from build123d import *

# Parameters (mm, degrees)
F0_R     = 47.2126506678
F0_R_2   = 20.2272154061
F1_DEPTH = 50.8
F2_R     = 3.175
F2_R_2   = 4.8238037601
F3_DEPTH = 50.801
F4_R     = 4.3834323194
F5_ANGLE = 180


# Not quite as in the source:
# - the program builds the solid bodies; features that only make, move or delete a surface that nothing else refers to are left out


with BuildPart() as f1:
    # F0 (on Front) → F1 (new body)
    with BuildSketch(Plane.XZ):
        Circle(F0_R)
        Circle(F0_R_2, mode=Mode.SUBTRACT)
    extrude(amount=F1_DEPTH)

    # F2 (on Front) → F3 (cut, through all)
    with BuildSketch(Plane.XZ):
        with Locations((0, 34.7616262734)):
            Circle(F2_R)
        with Locations((0, -35.3442244232)):
            Circle(F2_R_2)
    extrude(amount=F3_DEPTH, mode=Mode.SUBTRACT)

    # F4 (on Front) → F5 (revolve)
    with BuildSketch(Plane.XZ):
        with Locations((-34.811783582, 0)):
            Circle(F4_R)
    revolve(axis=Axis((0, 0, 1.5608235262), (0, 0, -1)), revolution_arc=F5_ANGLE)


solid = f1.part
Geometry check sheet. Reference: the model listing, model coordinates, mm. Round coordinates to 2 decimals unless told otherwise and drop trailing zeros. Write each loop counter-clockwise with the first axis right and the second up, starting at its lowest first coordinate (ties: lowest second). Pieces come first, ordered by that corner, then holes.
Item 1: Section check D-D (y = -36.5). Record the boundary of the cut face in (x, z) (3 decimals), plus the area to 3 significant figures.
Determined:
outline: circle Ø94.425 at (0, 0); hole circle Ø40.454 at (0, 0); hole circle Ø9.648 at (0, -35.344); hole circle Ø6.35 at (0, 34.762)
area: 5,610 mm2
Item 2: Section check A-A (z = -33). Record the boundary of the cut face in (x, y).
Determined:
outline: (-33.76, -50.8) - (-4.22, -50.8) - (-4.22, 0) - (-33.76, 0) - close; (4.22, -50.8) - (33.76, -50.8) - (33.76, 0) - (4.22, 0) - close
Item 3: Section check C-C (z = -16.5). Record the boundary of the cut face in (x, y), plus the area to 3 significant figures.
Determined:
outline: (-44.24, -50.8) - (-11.7, -50.8) - (-11.7, 0) - (-44.24, 0) - close; (11.7, -50.8) - (44.24, -50.8) - (44.24, 0) - (11.7, 0) - close
area: 3,310 mm2
Item 4: Go/stop test with flat-tipped pins: pin 1 Ø1.5 at (x, z) = (-20.5, 31) entering from +Y; pin 2 Ø2 at (y, z) = (-27, 8) entering from +X; pin 3 Ø4 at (y, z) = (-10, 25.5) entering from -X; pin 4 Ø12.5 at (x, z) = (0, -35.34) entering from -Y. Record where each tip stops, or that it passes through.
Determined:
pin 1: stops at y = 0
pin 2: stops at x = 46.69
pin 3: stops at x = -40.95
pin 4: stops at y = -50.8
Item 5: Material ranges on line 1 along Z through (x, y) = (0, -12); line 2 along Z through (x, y) = (2, -17); line 3 along Y through (x, z) = (-28, 34), recorded low to high.
Determined:
line 1: z = -47.21 to -40.17, -30.52 to -20.23, 20.23 to 31.59, 37.94 to 47.21
line 2: z = -47.17 to -39.73, -30.95 to -20.13, 20.13 to 32.3, 37.23 to 47.17
line 3: y = -50.8 to 0
Item 6: Section check B-B (x = 0). Record the boundary of the cut face in (y, z), plus the area to 3 significant figures.
Determined:
outline: (-50.8, -47.21) - (0, -47.21) - (0, -40.17) - (-50.8, -40.17) - close; (-50.8, -30.52) - (0, -30.52) - (0, -20.23) - (-50.8, -20.23) - close; (-50.8, 20.23) - (0, 20.23) - (0, 31.59) - (-50.8, 31.59) - close; (-50.8, 37.94) - (0, 37.94) - (0, 47.21) - (-50.8, 47.21) - close; circle Ø8.77 at (34.81, 0)
area: 1,990 mm2
Item 7: Mould release check, pull along X, two halves, no side actions. Record for faces 1 (the face through (10, -50.8, -20)), 2 (the face through (-4.385, -25.044, -19.746)), 3 (the face through (-6.15, -25.04, 46.81)), 4 (the face through (-0.688, -25.044, 31.662)): +X half, -X half, draft (parallel to the pull), parting line (faces both ways), or undercut.
Determined:
face 1: draft
face 2: undercut
face 3: parting line
face 4: undercut
